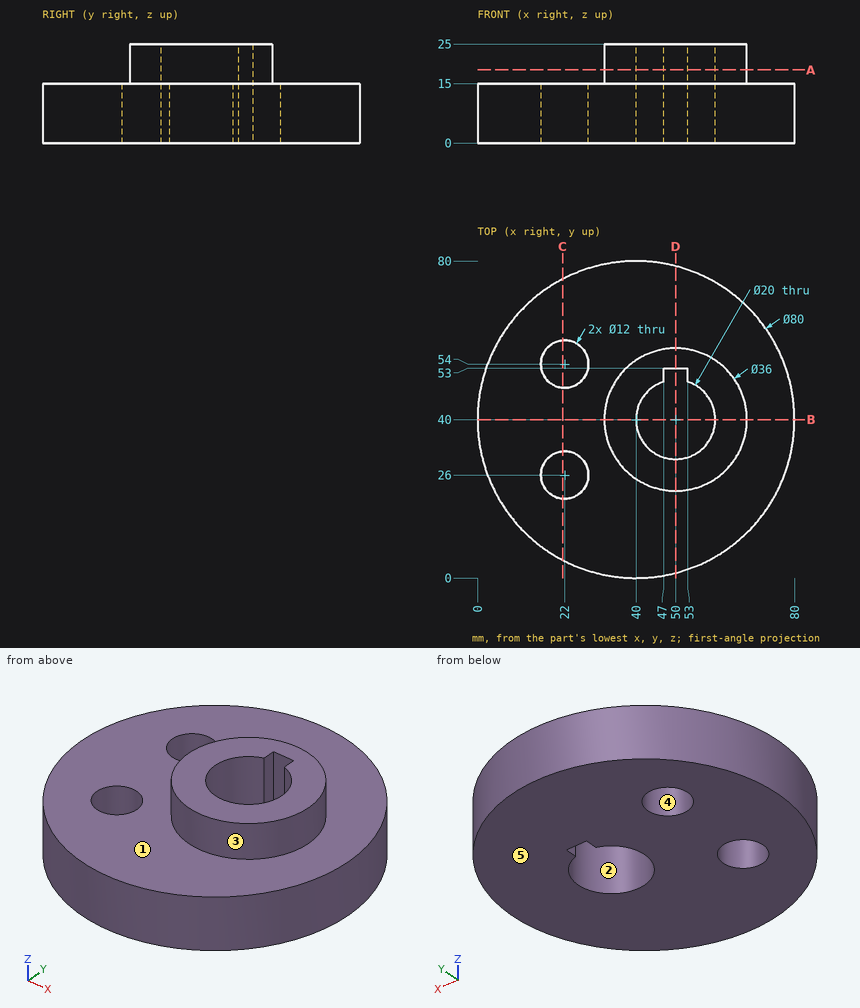
Can you work these out from the drawing? Everything is in mm from the part's minimum corner. A direction names the side the tool comes from. Round coordinates to 2 decimals unless told otherwise and drop trailing zeros. Loops run counter-clockwise (first coordinate to the right, second up) from the corner with the lowest first, then second, coordinate; pieces in that order, holes last. Notation, with made-up numbers: (60.5, 88.5) -> (67.5, 88.5) arc R21 cw to (67.5, 95.5) -> close; hole circle Ø6 at (16, -1.75). An arc over 180 degrees is marked (long way). Answer in a Markdown table with one row per item.
Item 1: Suppose I cut it at D-D, the plane x = 50. List the corners of the cut face in (y, z) for me, plus the area to 3 significant figures.
Answer block:
| item | result |
|---|---|
| outline | (1.27, 0) -> (30, 0) -> (30, 25) -> (22, 25) -> (22, 15) -> (1.27, 15) -> close; (53, 0) -> (78.73, 0) -> (78.73, 15) -> (58, 15) -> (58, 25) -> (53, 25) -> close |
| area | 947 mm² |
Item 2: Suppose I cut it at C-C, the plane x = 21.5. List the corners of the cut face in (y, z) for me.
Answer block:
| item | result |
|---|---|
| outline | (4.54, 0) -> (20.02, 0) -> (20.02, 15) -> (4.54, 15) -> close; (31.98, 0) -> (48.02, 0) -> (48.02, 15) -> (31.98, 15) -> close; (59.98, 0) -> (75.46, 0) -> (75.46, 15) -> (59.98, 15) -> close |
Item 3: Suppose I cut it at A-A, the plane z = 18.5. List the corners of the cut face in (x, y) for me.
Answer block:
| item | result |
|---|---|
| outline | circle Ø36 at (50, 40); hole (47, 49.54) arc R10 ccw (long way) to (53, 49.54) -> (53, 53) -> (47, 53) -> close |
Item 4: We'd pull the mould along X, two halves only. Please class the marked faces 3, 4 and 5: released by +X, released by -X, zero draft, split by the parting line, or undercut.
Answer block:
| item | result |
|---|---|
| face 3 | split by the parting line |
| face 4 | undercut |
| face 5 | zero draft |
Item 5: If I drill on probe 1 along Y at (x, z) = (22, 5); probe 2 along Z at (x, y) = (26, 42.5); probe 3 along X at (y, z) = (54, 8.25), over which ranges is the centre line in solid material (lowest first)?
Answer block:
| item | result |
|---|---|
| probe 1 | 4.28 to 20, 32 to 48, 60 to 75.72 |
| probe 2 | 0 to 15 |
| probe 3 | 2.53 to 16, 28 to 77.47 |
Item 6: Will these pins go through, and if not, where does the flat tip stop? P1, Ø1, axis at x = 72, z = 12, coming from the +Y side; P2, Ø3, axis at x = 49, z = 12.5, coming from the -Y side; P3, Ø4, axis at y = 52, z = 14, coming from the +X side.
Answer block:
| item | result |
|---|---|
| P1 | y = 64.65 |
| P2 | y = 0.71 |
| P3 | x = 78.73 |
Item 7: On a 3-axis mill with a long thin cutter (end or side, diameter ignored), from which of +Z, -Z, +X, -X, +Y, -Y can I reach the whole of each face in a straight line? I mean the marked faces 1 and 2. Say none if no direction works.
Answer block:
| item | result |
|---|---|
| face 1 | +Z |
| face 2 | +Z, -Z |
Item 8: Suppose I cut it at B-B, the plane y = 40. List the corners of the cut face in (x, z) for me, plus the area to 3 significant figures.
Answer block:
| item | result |
|---|---|
| outline | (0, 0) -> (40, 0) -> (40, 25) -> (32, 25) -> (32, 15) -> (0, 15) -> close; (60, 0) -> (80, 0) -> (80, 15) -> (68, 15) -> (68, 25) -> (60, 25) -> close |
| area | 1,060 mm² |
